Could you check a few things on this model? Use its own coordinates, in mm. Give positions to 0.01 mm unless a question says otherwise; leave off trailing zeros. Order: outer loops, then holes, each group sorted by start corner. A loop starts at its lowest first (then second) coordinate and runs counter-clockwise, first axis right, second up. Notation, with made-up numbers: M -30,20.5 L -13,20.5 A34 ccw -13,50.5 Z; hole C 30.5,55.5 d3. An arc over 180 degrees is marked long. Use a Markdown table: item, result. Add a question column.
```python
from build123d import *

# Parameters (mm, degrees)
SKETCH1_R      = 3.302
EXTRUDE1_DEPTH = 6.731


with BuildPart() as part:
    # Sketch1 → Extrude1 (new body)
    with BuildSketch(Plane(origin=(0, 0, 0), x_dir=(1, 0, 0), z_dir=(0, 1, 0))):
        Polygon((7.332348419, 0), (3.666174209, 6.35), (-3.666174209, 6.35), (-7.332348419, 0), (-3.666174209, -6.35), (3.666174209, -6.35), align=None)
        with Locations(Location((0, 0, 0), (0, 0, 270))):
            Circle(SKETCH1_R, mode=Mode.SUBTRACT)
    extrude(amount=EXTRUDE1_DEPTH)

    # Sketch2 → Cut-Revolve1 (revolve, cut)
    with BuildSketch(Plane.XY):
        with BuildLine():
            Line((6.35, 6.731), (7.332348419, 6.731))
            Line((7.332348419, 6.731), (7.332348419, 5.9055))
            ThreePointArc((7.332348419, 5.9055), (6.862078786, 6.343126533), (6.35, 6.731))
        make_face()
        with BuildLine():
            Line((7.332348419, 0), (7.332348419, 0.8255))
            ThreePointArc((7.332348419, 0.8255), (6.862078786, 0.387873467), (6.35, 0))
            Line((6.35, 0), (7.332348419, 0))
        make_face()
    revolve(axis=Axis((0, 0, 0), (0, 1, 0)), mode=Mode.SUBTRACT)


solid = part.part
```
1) For pin 1 (1 mm diameter, centred on x = 0, z = -3, fed in from +Y); pin 2 (5 mm diameter, centred on x = -0.5, z = 0.5, fed in from +Y); pin 3 (2 mm diameter, centred on x = -5, y = 4.5, fed in from +Z); pin 4 (1 mm diameter, centred on y = 2.5, z = -1, fed in from -X), each with a flat end and sliding along its axis, tell me the tip position at first contact or that it passes through.
2) Please list where these lines run through material, in increasing order: line 1 (Z direction, x = -2.75, y = 4); line 2 (Z direction, x = 0.25, y = 1.25); line 3 (X direction, y = 2.75, z = -1.5). Write a range as from..to.
3) We'd pull the mould along X, two halves only. Please class faces 1 (the face through (0.99, 3.32, 3.15)), 2 (the face through (-5.525, 3.318, 3.131)), 3 (the face through (0, 3, 6.35)): pulls with the +X half, pulls with the -X half, needs draft (parallel to the pull), parting line crosses it, or undercut.
4) Suppose I cut it at A-A on y = 4. Please give me the cut outline in (x, z).
Values found:
| question | item | result |
|---|---|---|
| 1 | pin 1 | stops at y = 6.73 |
| 1 | pin 2 | passes through |
| 1 | pin 3 | stops at z = 5.77 |
| 1 | pin 4 | stops at x = -7.04 |
| 2 | line 1 | z = -6.35..-1.83, 1.83..6.35 |
| 2 | line 2 | z = -6.35..-3.29, 3.29..6.35 |
| 2 | line 3 | x = -6.47..-2.94, 2.94..6.47 |
| 3 | face 1 | undercut |
| 3 | face 2 | pulls with the -X half |
| 3 | face 3 | needs draft |
| 4 | outline | M -7.33,0 L -3.67,-6.35 L 3.67,-6.35 L 7.33,0 L 3.67,6.35 L -3.67,6.35 Z; hole C 0,0 d6.6 |
